```python
from build123d import *

# Parameters (mm, degrees)
F0_R     = 7.62
F1_DEPTH = 43.18
F3_DEPTH = 5.08
F4_R     = 2.54


with BuildPart() as f1:
    # F0 (on Front) → F1 (new body)
    with BuildSketch(Plane.XZ):
        Circle(F0_R)
    extrude(amount=-F1_DEPTH)

    # F2 (on face) → F3 (cut)
    with BuildSketch(Plane(origin=(0, 43.18, 0), x_dir=(-1, 0, 0), z_dir=(0, 1, 0))):
        with BuildLine():
            Line((-1.863431, -7.388642), (-1.863431, 7.388642))
            ThreePointArc((-1.863431, 7.388642), (-7.62, 0), (-1.863431, -7.388642))
        make_face()
    extrude(amount=-F3_DEPTH, mode=Mode.SUBTRACT)

    # F4
    f4_edges = [f1.edges().sort_by_distance(p)[0] for p in [
        (-7.62, 43.18, 0),
    ]]
    fillet(f4_edges, radius=F4_R)


solid = f1.part
```
Here's how the part is built. I have some questions about the finished solid (model axes, mm). A direction names the side the tool comes from. Coordinates: 2 decimals unless noted, no trailing zeros. Loops run counter-clockwise (first coordinate to the right, second up) from the corner with the lowest first, then second, coordinate; pieces in that order, holes last. Notation, with made-up numbers: (80.25, 5.5) - (123.25, 5.5) arc R20 ccw to (123.25, 38.5) - close; hole circle Ø4 at (60.25, 31). An arc over 180 degrees is marked (long way). Return JSON: item names as keys, results as strings. Group by question number.
Item 1: If we section it at A-A on z = 0: Write out the boundary of the cut face in (x, y).
Item 2: Will these pins go through, and if not, where does the flat tip stop? P1, Ø5.5, axis at y = 41, z = -3, coming from the +X side; P2, Ø1.5, axis at y = 28, z = 3.5, coming from the -X side; P3, Ø3, axis at y = 22.5, z = 2.5, coming from the -X side.
Item 3: If we section it at B-B on y = 26: Write out the boundary of the cut face in (x, z).
Item 4: On a 3-axis mill with a long thin cutter (end or side, diameter ignored), from which of +Z, -Z, +X, -X, +Y, -Y can I reach the whole of each face in a straight line? I mean faces 1 (the face through (0, 0, 0)), 2 (the face through (1.863, 41, 0)). Say none if no direction works.
Item 5: I need wall thicknesses on line 1 (Y direction, x = 5, z = 4); line 2 (Z direction, x = 7, y = 28.5); line 3 (Z direction, x = -1.5, y = 14). Which ranges of each line are inside material? Lowest first, please. Write a range as from..to.
Calculated:
{
 "1": {"outline": "(-7.62, 0) - (7.62, 0) - (7.62, 38.1) - (1.86, 38.1) - (1.86, 43.18) - (-5.08, 43.18) arc R2.54 ccw to (-7.62, 40.64) - close"},
 "2": {"P1": "stops at x = 1.86", "P2": "stops at x = -7.11", "P3": "stops at x = -7.55"},
 "3": {"outline": "circle Ø15.24 at (0, 0)"},
 "4": {"face 1": "+Z, -Z, +X, -X, -Y", "face 2": "+Z, -Z, +X, +Y"},
 "5": {"line 1": "y = 0..38.1", "line 2": "z = -3.01..3.01", "line 3": "z = -7.47..7.47"}
}
